Check sheet for the modelled part. Datum: model origin and axes. Units: mm. Give positions to 0.01 mm unless a question says otherwise; leave off trailing zeros. Loops run counter-clockwise (first coordinate to the right, second up) from the corner with the lowest first, then second, coordinate; pieces in that order, holes last. Notation, with made-up numbers: (86, -29) - (130, -29) arc R22 cw to (130, 2) - close; hole circle Ø4 at (71, -16.75). An arc over 180 degrees is marked (long way). Answer in a Markdown table with one row per item. Add a question column.
(1) Thickness scan on L1, parallel to Z at x = -0.25, y = 3; L2, parallel to X at y = -3, z = 102; L3, parallel to X at y = -3.5, z = 37. Record the ranges inside material, lowest first.
(2) Sectioned sample at A-A on z = 68. Enter the section's corners in (x, y), then the cut area to 3 significant figures.
(3) Go/stop test with flat-tipped pins: P1, Ø2, axis at x = -3, z = 95, coming from the -Y side; P2, Ø1, axis at y = 2.5, z = 33, coming from the -X side; P3, Ø4, axis at y = 2.5, z = 100, coming from the -X side. Record where each tip stops, or that it passes through.
from build123d import *

# Parameters (mm, degrees)
CYLINDER_R      = 4
CYLINDER_DEPTH  = 150
CHAMFER_SIZE    = 1
CHAMFER001_SIZE = 1


with BuildPart() as part:
    # Cylinder → Cylinder (new body)
    with BuildSketch(Plane.XY):
        Circle(CYLINDER_R)
    extrude(amount=CYLINDER_DEPTH)

    # Chamfer
    chamfer_edges = [part.edges().sort_by_distance(p)[0] for p in [
        (-4, 0, 150),
    ]]
    chamfer(chamfer_edges, length=CHAMFER_SIZE)

    # Chamfer001
    chamfer001_edges = [part.edges().sort_by_distance(p)[0] for p in [
        (-4, 0, 0),
    ]]
    chamfer(chamfer001_edges, length=CHAMFER001_SIZE)


solid = part.part
Reply:
| question | item | result |
|---|---|---|
| 1 | L1 | 0.01 to 149.99 |
| 1 | L2 | -2.65 to 2.65 |
| 1 | L3 | -1.94 to 1.94 |
| 2 | outline | circle Ø8 at (0, 0) |
| 2 | area | 50.3 mm^2 |
| 3 | P1 | y = -3.46 |
| 3 | P2 | x = -3.46 |
| 3 | P3 | x = -3.97 |
